Work out the finished part from the listing and answer in its coordinate system (mm). A direction names the side the tool comes from. Coordinates: 2 decimals unless noted, no trailing zeros. Write each loop counter-clockwise with the first axis right and the second up, starting at its lowest first coordinate (ties: lowest second). Pieces come first, ordered by that corner, then holes. Notation, with made-up numbers: (29, 8) - (82, 8) arc R26 cw to (82, 25) - close; hole circle Ø1 at (-11, -22). An arc over 180 degrees is marked (long way). One line per item, written item: value.
```python
from build123d import *

# Parameters (mm, degrees)
F0_R     = 63.5
F1_DEPTH = 254
F2_SIZE2 = 5.08
F2_SIZE  = 5.08
F4_D     = 6.35
F5_DEPTH = 122.428


with BuildPart() as f1:
    # F0 (on Front) → F1 (new body)
    with BuildSketch(Plane.XZ):
        Circle(F0_R)
    extrude(amount=-F1_DEPTH)

    # F2
    f2_edges = [f1.edges().sort_by_distance(p)[0] for p in [
        (63.5, 127, 0),
        (-63.5, 0, 0),
        (-63.5, 254, 0),
    ]]
    chamfer(f2_edges, length=F2_SIZE, length2=F2_SIZE2)

    # F4 (through all)
    with Locations(Plane(origin=(0, 254, 0), x_dir=(-1, 0, 0), z_dir=(0, 1, 0))):
        with Locations((0, 0)):
            Hole(F4_D / 2)

    # F5 (add): a face of the model
    f5_faces = [f1.faces().sort_by_distance(p)[0] for p in [
        (-56.7676328737, 0, 0),
    ]]
    extrude(f5_faces, amount=F5_DEPTH)


solid = f1.part
```
Item 1: Section B-B, the plane y = 186 is taken. Determine the outline of the cut face in (x, z) (3 decimals), then the cut area to 3 significant figures.
Evaluation:
outline: circle Ø127 at (0, 0); hole circle Ø6.35 at (0, 0)
area: 12,600 mm2
Item 2: Given pin 1 (6 mm diameter, centred on y = 170.5, z = 7.5, fed in from -X); pin 2 (10 mm diameter, centred on x = -5, y = 95, fed in from -Z); pin 3 (1.5 mm diameter, centred on x = 17, y = -17.5, fed in from +Z), each flat-ended and moving along its own axis, determine where each tip first touches the part or whether it passes through.
Evaluation:
pin 1: stops at x = -63.34
pin 2: stops at z = -63.5
pin 3: stops at z = 56.11
Item 3: Consider probe 1 along Z at (x, y) = (0, 60) (3 decimals); probe 2 along Z at (x, y) = (0, -92.5) (3 decimals); probe 3 along X at (y, z) = (3, 2). Determine where each line is inside the solid, lowest interval first.
Evaluation:
probe 1: z = -63.5 to -3.175, 3.175 to 63.5
probe 2: z = -58.42 to -3.175, 3.175 to 58.42
probe 3: x = -61.39 to -2.47, 2.47 to 61.39
Item 4: Section A-A, the plane y = -47 is taken. Determine the outline of the cut face in (x, z) (3 decimals), then the cut area to 3 significant figures.
Evaluation:
outline: circle Ø116.84 at (0, 0); hole circle Ø6.35 at (0, 0)
area: 10,700 mm2
Item 5: Which of the six approach directions +Z, -Z, +X, -X, +Y, -Y give full straight-line access (tool end or side, diameter ignored) to faces 1 (the face through (-13.77, 125.29, -61.99)), 2 (the face through (-43.06, -60.36, 39.48))?
Evaluation:
face 1: +Y, -Y
face 2: -Y
